Source: CAD feature listing. Evaluate the final solid. Frame: model axes, mm. A direction names the side the tool comes from. Coordinates: 2 decimals unless noted, no trailing zeros. Write each loop counter-clockwise with the first axis right and the second up, starting at its lowest first coordinate (ties: lowest second). Pieces come first, ordered by that corner, then holes. Notation, with made-up numbers: M 7,15 L 33,15 A33 ccw 33,46 Z; hole C 57,14.25 d1. An arc over 180 degrees is marked long. One line per item, written item: value. Start each with the question number.
Item 1: Set-up query: faces 1 (the cylindrical face through (-3, 0, 64)), 2 (the flat face through (0, 0, 0)), 3 (the flat face through (4, 0, 160)). Return all of +Z, -Z, +X, -X, +Y, -Y with unobstructed straight access to the full face (end or side cutting, diameter ignored); none if empty.
Item 2: Pin query (flat end, axial travel): P1, Ø12, axis at x = 0, z = 29.5, coming from the +Y side; P2, Ø4, axis at x = -63.5, y = 75.5, coming from the +Z side; P3, Ø12, axis at x = -61.5, y = -2, coming from the +Z side. Return the tip coordinate at first contact, or that it passes through.
Item 3: Cut plane A-A, the plane z = 53. Output: boundary loops of the cut face in (x, y).
Item 4: Ray query, L1, parallel to Z at x = -54, y = -0.5; L2, parallel to Z at x = 62, y = -58. Return the intervals inside material, ascending. Write a range as from..to.
Item 5: Cut plane B-B, the plane z = 146. Output: boundary loops of the cut face in (x, y), then the cut area to 3 significant figures.
```python
from build123d import *

# Parameters (mm, degrees)
F0_R     = 3
F1_DEPTH = 130
F2_R     = 100
F2_R_2   = 3
F3_DEPTH = 30
F4_SIZE2 = 29
F4_SIZE  = 90
F5_R     = 3.4961547094
F6_DEPTH = 7.6


# Not quite as in the source:
# - a fillet or chamfer that OpenCascade refuses, or shapes differently, is made with other operations: its cross-section is extruded or revolved along the edge and cut away or added


with BuildPart() as f1:
    # F0 (on Top) → F1 (new body)
    with BuildSketch(Plane.XY):
        Circle(F0_R)
    extrude(amount=F1_DEPTH)

    # F2 (on face) → F3 (join)
    with BuildSketch(Plane.XY.offset(130)):
        Circle(F2_R)
        Circle(F2_R_2, mode=Mode.SUBTRACT)
        Circle(F2_R_2)
    extrude(amount=F3_DEPTH)

    # F4
    f4_edges = [f1.edges().sort_by_distance(p)[0] for p in [
        (-100, 0, 160),
    ]]
    f4_side = f1.faces().sort_by_distance((0, 0, 160))[0]
    chamfer(f4_edges, length=F4_SIZE, length2=F4_SIZE2, reference=f4_side)

    # F5 (on face) → F6 (join)
    with BuildSketch(Plane.XY.offset(160)):
        Circle(F5_R)
    extrude(amount=F6_DEPTH)

    # F7: chamfer of 1 x 10 on 1 edges, made by hand


with BuildPart() as f7_tool2:
    # F7_s3 → F7_t4 (revolve)
    with BuildSketch(Plane.XZ):
        Polygon((3.4961547094, 157.6), (2.4961547094, 167.6), (3.4961547094, 167.6), align=None)
    revolve(axis=Axis((0, 0, 167.6), (0, 0, 1)))

    split(bisect_by=Plane.XY.offset(160), keep=Keep.TOP)


with BuildPart() as f1_1:
    add(f1.part)

    # F7_t1: cut F7_tool2
    add(f7_tool2.part, mode=Mode.SUBTRACT)


solid = f1_1.part
```
From the geometry:
1. face 1: -Z
1. face 2: -Z, +X, -X, +Y, -Y
1. face 3: +Z
2. P1: stops at y = 3
2. P2: stops at z = 132.08
2. P3: stops at z = 145.33
3. outline: C 0,0 d6
4. L1: z = 130..145.82
4. L2: z = 130..135.87
5. outline: C 0,0 d106.9
5. area: 8,970 mm²
